from build123d import *

# Parameters (mm, degrees)
BOSS_EXTRUDE1_DEPTH = 12
SKETCH4_W           = 76.386919113
SKETCH4_H           = 24
SKETCH4_R           = 4
BOSS_EXTRUDE2_DEPTH = 12
SKETCH4_3_R         = 8
SKETCH4_3_R_2       = 4
CUT_EXTRUDE1_DEPTH  = 5.15
FILLET1_R           = 12
SKETCH5_R           = 1.7
CUT_EXTRUDE2_DEPTH  = 123.426024465
CUT_EXTRUDE3_START  = -5
SKETCH5_3_R         = 3
CUT_EXTRUDE3_DEPTH  = 118.426024512


with BuildPart() as part:
    # Sketch3 → Boss-Extrude1 (new body)
    with BuildSketch(Plane(origin=(0, 0, 0), x_dir=(1, 0, 0), z_dir=(0, 1, 0))):
        with BuildLine():
            Line((-26, 15.011106999), (0, 30.022213998))
            Line((0, 30.022213998), (26, 15.011106999))
            Line((26, 15.011106999), (26, 12))
            Line((26, 12), (31.811947441, 12))
            ThreePointArc((31.811947441, 12), (-34, 0), (31.811947441, -12))
            Line((31.811947441, -12), (26, -12))
            Line((26, -12), (26, -15.011106999))
            Line((26, -15.011106999), (0, -30.022213998))
            Line((0, -30.022213998), (-26, -15.011106999))
            Line((-26, -15.011106999), (-26, 15.011106999))
        make_face()
        with BuildLine():
            Line((31.811947441, 12), (26, 12))
            Line((26, 12), (26, -12))
            Line((26, -12), (31.811947441, -12))
            ThreePointArc((31.811947441, -12), (33.448514264, -6.098925602), (34, 0))
            ThreePointArc((34, 0), (33.448514264, 6.098925602), (31.811947441, 12))
        make_face()
        with BuildLine():
            Line((47.8, 12), (31.811947441, 12))
            ThreePointArc((31.811947441, 12), (33.448514264, 6.098925602), (34, 0))
            ThreePointArc((34, 0), (33.448514264, -6.098925602), (31.811947441, -12))
            Line((31.811947441, -12), (47.8, -12))
            Line((47.8, -12), (47.8, 12))
        make_face()
    extrude(amount=BOSS_EXTRUDE1_DEPTH)

    # Sketch4 → Boss-Extrude2 (add)
    with BuildSketch(Plane(origin=(23.9, -23.9, 0), x_dir=(0.7071067811865462, 0.707106781186549, 0), z_dir=(0.707106781186549, -0.7071067811865462, 0))):
        with Locations((71.993163698, 0)):
            Rectangle(SKETCH4_W, SKETCH4_H)
        with Locations((94.186623254, 0)):
            Circle(SKETCH4_R, mode=Mode.SUBTRACT)
    extrude(amount=-BOSS_EXTRUDE2_DEPTH)

    # Sketch4<3> → Cut-Extrude1 (cut)
    with BuildSketch(Plane(origin=(23.9, -23.9, 0), x_dir=(0.7071067811865462, 0.707106781186549, 0), z_dir=(0.707106781186549, -0.7071067811865462, 0))):
        with Locations((94.186623254, 0)):
            Circle(SKETCH4_3_R)
        with Locations((94.186623254, 0)):
            Circle(SKETCH4_3_R_2, mode=Mode.SUBTRACT)
    extrude(amount=-CUT_EXTRUDE1_DEPTH, mode=Mode.SUBTRACT)

    # Fillet1
    fillet1_edges = [part.edges().sort_by_distance(p)[0] for p in [
        (97.571067812, 58.256349186, -12),
        (97.571067812, 58.256349186, 12),
    ]]
    fillet(fillet1_edges, radius=FILLET1_R - 0.0001)  # a hair under: the kernel refuses the full size

    # Sketch5 → Cut-Extrude2 (cut, through all)
    with BuildSketch(Plane(origin=(13, 0, -22.516660498), x_dir=(0.8660254037844415, 0, 0.4999999999999951), z_dir=(-0.49999999999999517, 0, 0.8660254037844416))):
        with Locations((0, 6)):
            Circle(SKETCH5_R)
    cut_extrude2 = extrude(amount=-CUT_EXTRUDE2_DEPTH, mode=Mode.SUBTRACT)

    # Sketch5<3> → Cut-Extrude3 (cut, through all)
    with BuildSketch(Plane(origin=(13, 0, -22.516660498), x_dir=(0.8660254037844415, 0, 0.4999999999999951), z_dir=(-0.49999999999999517, 0, 0.8660254037844416)).offset(CUT_EXTRUDE3_START)):
        with Locations((0, 6)):
            Circle(SKETCH5_3_R)
    cut_extrude3 = extrude(amount=-CUT_EXTRUDE3_DEPTH, mode=Mode.SUBTRACT)

    # Mirror1: Cut-Extrude2, Cut-Extrude3 across plane
    add(cut_extrude2.mirror(Plane(origin=(0, 0, 0), x_dir=(0.8660254037844415, 0, 0.49999999999999517), z_dir=(-0.49999999999999506, 0, 0.8660254037844415))), mode=Mode.SUBTRACT)
    add(cut_extrude3.mirror(Plane(origin=(0, 0, 0), x_dir=(0.8660254037844415, 0, 0.49999999999999517), z_dir=(-0.49999999999999506, 0, 0.8660254037844415))), mode=Mode.SUBTRACT)


solid = part.part
Input: part model. Units: mm. Frame: model coordinates. A direction names the side the tool comes from. Coordinates: 2 decimals unless noted, no trailing zeros. Loops run counter-clockwise (first coordinate to the right, second up) from the corner with the lowest first, then second, coordinate; pieces in that order, holes last. Notation, with made-up numbers: (-25, -21.5) -> (17, -21.5) arc R20 cw to (17, -1.5) -> close; hole circle Ø11 at (25.5, 27.25). An arc over 180 degrees is marked (long way). Write each question's results on one line, items separated by ' | '. Start each with the question number.
Q1. Pull-direction query (Y, two-part tool) for faces 1 (the flat face through (67.73, 36.9, 0.17)), 2 (the flat face through (-15.536, 4.042, 26.826)), 3 (the flat face through (26, 6, 0)); classes: released by +Y, released by -Y, zero draft, split by the parting line, or undercut.
Q2. Pin query (flat end, axial travel): pin 1 (5 mm diameter, centred on x = 69, z = 1.5, fed in from -Y); pin 2 (1.5 mm diameter, centred on x = 62, z = -5.5, fed in from -Y); pin 3 (16 mm diameter, centred on x = 76.5, y = 19, fed in from -Z). Return the tip coordinate at first contact, or that it passes through.
Q3. Section A-A, the plane x = -4.5. Return the cut outline in (y, z).
Q4. Section C-C, the plane y = 31. Return the cut outline in (x, z), plus the area to 3 significant figures.
Q5. Ray query, line 1 (Y direction, x = 35, z = 11); line 2 (X direction, y = 9.5, z = -10.5); line 3 (X direction, y = 36, z = 7.5). Return the intervals inside material, ascending. Write a range as from..to.
Q6. Section B-B, the plane x = 36. Return the cut outline in (y, z), plus the area to 3 significant figures.
Q7. Reachability of faces 4 (the flat face through (61, 24, -12)), 5 (the flat face through (60, 25, 12)), 6 (the flat face through (89.293, 48.777, -3.444)), 7 (the flat face through (-12.82, 3.25, 22.62)) from +Z, -Z, +X, -X, +Y, -Y: full face, straight path, thin tool, end or side. Return the list, or none.
Found:
1) face 1: released by +Y | face 2: undercut | face 3: zero draft
2) pin 1: y = 18.7 | pin 2: y = 13.45 | pin 3: z = -12
3) outline: (0, -33.7) -> (12, -33.7) -> (12, -27.42) -> (0, -27.42) -> close; (0, 27.42) -> (12, 27.42) -> (12, 33.7) -> (0, 33.7) -> close
4) outline: (61.83, -12) -> (78.8, -12) -> (78.8, 12) -> (61.83, 12) -> close | area: 407 mm2
5) line 1: 0..12 | line 2: -32.34..-26, 26..57.3 | line 3: 66.83..83.8
6) outline: (0, -12) -> (12, -12) -> (12, 12) -> (0, 12) -> close | area: 288 mm2
7) face 4: -Z, +X, +Y, -Y | face 5: +Z, +X, +Y, -Y | face 6: none | face 7: +Y, -Y
